Job drawing, mm, ordinate dimensions from the low corner. One solid piece. A direction names the side the tool comes from. Give positions to 0.01 mm unless a question says otherwise; leave off trailing zeros. Write each loop counter-clockwise with the first axis right and the second up, starting at its lowest first coordinate (ties: lowest second). Pieces come first, ordered by that corner, then holes. Notation, with made-up numbers: (82, 47) -> (123, 47) arc R21 ccw to (123, 66) -> close; hole circle Ø1 at (20, 65.5). An arc over 180 degrees is marked (long way). One line per question, with ' | ' between items. Start each with the question number.
(1) Band-saw the part on D-D, the plane z = 12.5. Give the cut face in (x, y).
(2) Pull direction X, two halves, no side cores. Call the marked faces 1, 2, 3 and 4: released by +X, released by -X, zero draft, split by the parting line, or undercut.
(3) Band-saw the part on A-A, the plane z = 1.5. Give the cut face in (x, y), and give its area (3 significant figures).
(4) Tool access for the marked faces 5, 6, 7 and 8: list every direction of +Z, -Z, +X, -X, +Y, -Y with a clear straight run to the whole face (end or side of a thin tool).
(5) Band-saw the part on C-C, the plane x = 5.2. Give the cut face in (y, z), and give its area (3 significant figures).
(6) Drill centre lines: probe 1 along X at (y, z) = (51.85, 14.5); probe 2 along Y at (x, z) = (5, 13); probe 3 along Y at (x, z) = (79.3, 4.5). Where is each one in solid material? Low to high. Write a range as from..to.
(7) Pin check, flat tips, straight feed: P1, Ø4, axis at x = 78, y = 6, coming from the +Z side; P2, Ø1, axis at x = 31.5, y = 19.5, coming from the +Z side; P3, Ø4, axis at x = 5.2, y = 51.85, coming from the -Z side; P4, Ø2.5, axis at y = 35.5, z = 5.5, coming from the -X side. Stop position of each tip, or through.
(8) Band-saw the part on B-B, the plane y = 5.15. Give the cut face in (x, z).
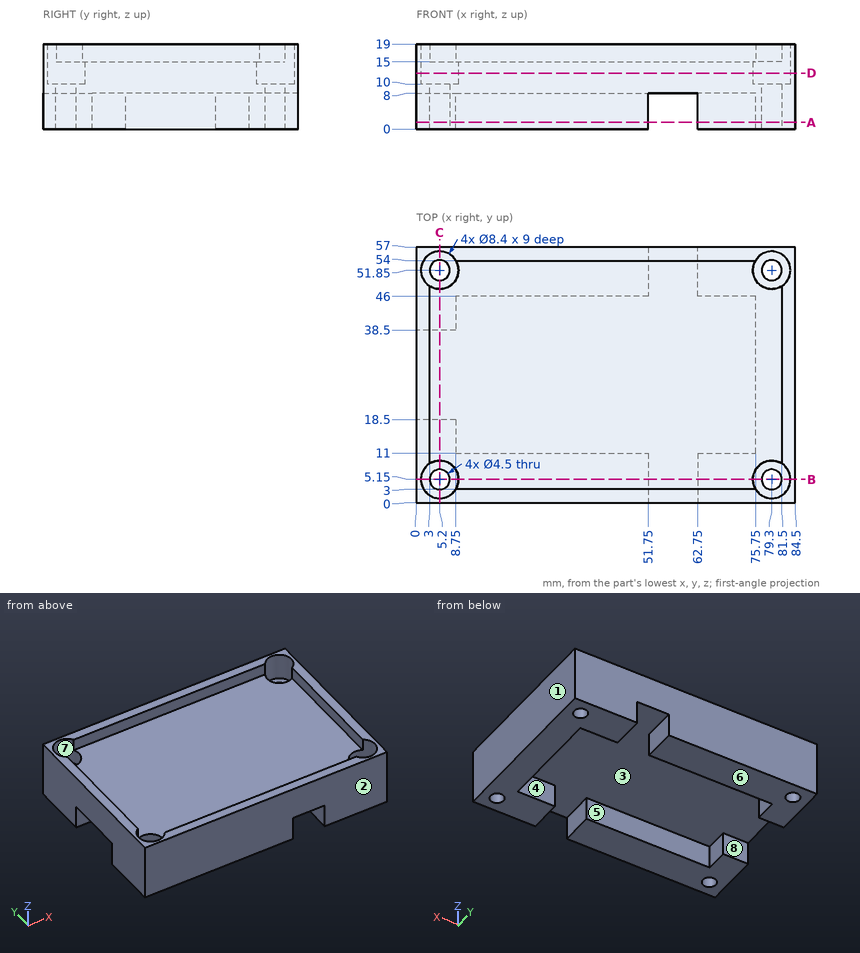
Results:
1) outline: (0, 0) -> (84.5, 0) -> (84.5, 57) -> (0, 57) -> close; hole circle Ø8.4 at (5.2, 5.15); hole circle Ø8.4 at (5.2, 51.85); hole circle Ø8.4 at (79.3, 5.15); hole circle Ø8.4 at (79.3, 51.85)
2) face 1: released by +X | face 2: zero draft | face 3: undercut | face 4: undercut
3) outline: (0, 0) -> (51.75, 0) -> (51.75, 11) -> (8.75, 11) -> (8.75, 18.5) -> (0, 18.5) -> close; (0, 38.5) -> (8.75, 38.5) -> (8.75, 46) -> (51.75, 46) -> (51.75, 57) -> (0, 57) -> close; (62.75, 0) -> (84.5, 0) -> (84.5, 57) -> (62.75, 57) -> (62.75, 46) -> (75.75, 46) -> (75.75, 11) -> (62.75, 11) -> close; hole circle Ø4.5 at (5.2, 5.15); hole circle Ø4.5 at (5.2, 51.85); hole circle Ø4.5 at (79.3, 5.15); hole circle Ø4.5 at (79.3, 51.85) | area: 1,990 mm²
4) face 5: -Z | face 6: -Z, +X, -X, +Y, -Y | face 7: +Z | face 8: -Z, -X
5) outline: (0, 0) -> (2.9, 0) -> (2.9, 10) -> (0.95, 10) -> (0.95, 19) -> (0, 19) -> close; (7.4, 0) -> (18.5, 0) -> (18.5, 8) -> (38.5, 8) -> (38.5, 0) -> (49.6, 0) -> (49.6, 10) -> (47.65, 10) -> (47.65, 15) -> (9.35, 15) -> (9.35, 10) -> (7.4, 10) -> close; (54.1, 0) -> (57, 0) -> (57, 19) -> (56.05, 19) -> (56.05, 10) -> (54.1, 10) -> close | area: 529 mm²
6) probe 1: x = 0..1, 9.4..75.1, 83.5..84.5 | probe 2: y = 0..0.95, 9.35..47.65, 56.05..57 | probe 3: y = 0..2.9, 7.4..49.6, 54.1..57
7) P1: stops at z = 10 | P2: stops at z = 15 | P3: passes through | P4: stops at x = 75.75
8) outline: (0, 0) -> (2.95, 0) -> (2.95, 10) -> (1, 10) -> (1, 19) -> (0, 19) -> close; (7.45, 0) -> (51.75, 0) -> (51.75, 8) -> (62.75, 8) -> (62.75, 0) -> (77.05, 0) -> (77.05, 10) -> (75.1, 10) -> (75.1, 15) -> (9.4, 15) -> (9.4, 10) -> (7.45, 10) -> close; (81.55, 0) -> (84.5, 0) -> (84.5, 19) -> (83.5, 19) -> (83.5, 10) -> (81.55, 10) -> close
